```python
from build123d import *

# Parameters (mm, degrees)
BOSS_EXTRUDE1_DEPTH = 63.5
BOSS_EXTRUDE2_DEPTH = 63.5
SKETCH6_R           = 12.254243907
CUT_EXTRUDE1_DEPTH  = 20.05
CUT_EXTRUDE2_DEPTH  = 19.05


with BuildPart() as part:
    # Sketch3 → Boss-Extrude1 (new body)
    with BuildSketch(Plane(origin=(0, 0, 0), x_dir=(1, 0, 0), z_dir=(0, 1, 0))):
        Polygon((-130.754517968, 4.672099354), (-130.754517968, -58.827900646), (-67.254517968, -58.827900646), (-67.254517968, -39.777900646), (-111.704517968, -39.777900646), (-111.704517968, 4.672099354), align=None)
    extrude(amount=BOSS_EXTRUDE1_DEPTH)

    # Sketch4 → Boss-Extrude2 (add)
    with BuildSketch(Plane(origin=(0, 0, -4.672099354), x_dir=(-1, 0, 0), z_dir=(0, 0, -1))):
        Polygon((130.754517968, 63.5), (130.754517968, 44.443431663), (175.135531737, 44.443431663), (175.135531737, 0), (194.183522013, 0), (194.183522013, 63.5), align=None)
    extrude(amount=-BOSS_EXTRUDE2_DEPTH)

    # Sketch6 → Cut-Extrude1 (cut, through all)
    with BuildSketch(Plane(origin=(0, 0, 39.777900646), x_dir=(-1, 0, 0), z_dir=(0, 0, -1))):
        with Locations((86.304517968, 31.75)):
            Circle(SKETCH6_R)
    extrude(amount=-CUT_EXTRUDE1_DEPTH, mode=Mode.SUBTRACT)

    # Sketch8 → Cut-Extrude2 (cut)
    with BuildSketch(Plane(origin=(-111.704517968, 0, 0), x_dir=(0, 0, -1), z_dir=(1, 0, 0))):
        Polygon((4.672099354, 0), (4.672099354, 25.326198551), (-20.654099197, 0), align=None)
    extrude(amount=-CUT_EXTRUDE2_DEPTH, mode=Mode.SUBTRACT)


solid = part.part
```
Read the model definition and answer for the solid it produces. Units are mm, in the model's axes. A direction names the side the tool comes from. Give positions to 0.01 mm unless a question says otherwise; leave off trailing zeros. Order: outer loops, then holes, each group sorted by start corner. A loop starts at its lowest first (then second) coordinate and runs counter-clockwise, first axis right, second up.
(1) Straight lines are drawn through the part: L1, parallel to X at y = 12.5, z = 48; L2, parallel to X at y = 32.5, z = 7; L3, parallel to Y at x = -135, z = 30. For each, find the intervals that lie inside material, in ascending order.
(2) Find section C-C (y = 15.5). Give the vertices of the cut face in (x, z).
(3) Find section D-D (x = -113). Give the vertices of the cut face in (y, z), plus the area to 3 significant figures.
(4) Given pin 1 (13.5 mm diameter, centred on x = -148.5, z = 35.5, fed in from -Y); pin 2 (1.5 mm diameter, centred on y = 36, z = 34.5, fed in from +X), each flat-ended and moving along its own axis, determine where each tip first touches the part or whether it passes through.
(5) For a pull along X with two mould halves and no side action, classify faces 1 (the flat face through (-111.705, 31, 18)), 2 (the flat face through (-175.136, 23, 27)), 3 (the flat face through (-194.184, 31, 27)), 4 (the cylindrical face through (-74.062, 32.289, 49.17)) as released by +X, released by -X, zero draft, split by the parting line, or undercut.
(6) Find section A-A (y = 31.75). Give the vertices of the cut face in (x, z).
(7) Find section B-B (z = 46). Give the vertices of the cut face in (x, y).
(8) For faces 5 (the flat face through (-99, 31, 39.778)), 6 (the flat face through (-121.096, 12.84, 7.814)), 7 (the flat face through (-153, 44.443, 27)), 8 (the flat face through (-107, 0, 44)), determine the directions among +Z, -Z, +X, -X, +Y, -Y from which every point of the face is accessible in a straight line to the end or side of a thin tool.
Result sheet:
1. L1: x = -194.18 to -175.14, -130.75 to -67.25
1. L2: x = -194.18 to -175.14, -130.75 to -111.7
1. L3: y = 44.44 to 63.5
2. outline: (-194.18, -4.67) - (-175.14, -4.67) - (-175.14, 58.83) - (-194.18, 58.83) - close; (-130.75, 5.15) - (-111.7, 5.15) - (-111.7, 39.78) - (-67.25, 39.78) - (-67.25, 58.83) - (-130.75, 58.83) - close
3. outline: (0, 20.65) - (25.33, -4.67) - (63.5, -4.67) - (63.5, 58.83) - (0, 58.83) - close
3. area: 3,710 mm2
4. pin 1: stops at y = 44.44
4. pin 2: stops at x = -111.7
5. face 1: released by +X
5. face 2: undercut
5. face 3: released by -X
5. face 4: undercut
6. outline: (-194.18, -4.67) - (-175.14, -4.67) - (-175.14, 58.83) - (-194.18, 58.83) - close; (-130.75, -4.67) - (-111.7, -4.67) - (-111.7, 39.78) - (-98.56, 39.78) - (-98.56, 58.83) - (-130.75, 58.83) - close; (-74.05, 39.78) - (-67.25, 39.78) - (-67.25, 58.83) - (-74.05, 58.83) - close
7. outline: (-194.18, 0) - (-175.14, 0) - (-175.14, 44.44) - (-130.75, 44.44) - (-130.75, 0) - (-67.25, 0) - (-67.25, 63.5) - (-194.18, 63.5) - close; hole circle Ø24.51 at (-86.3, 31.75)
8. face 5: -Z, +X, +Y, -Y
8. face 6: -Z, +X, -Y
8. face 7: +Z, -Z, -Y
8. face 8: +Z, -Z, +X, -X, -Y
